from build123d import *

# Parameters (mm, degrees)
F0_W     = 49
F0_H     = 20
F0_W_2   = 5
F0_H_2   = 33
F0_H_3   = 28
F0_H_4   = 5
F0_W_3   = 26.6433528662
F0_W_4   = 30
F0_R     = 3
F1_DEPTH = 3


# Not quite as in the source:
# - a feature names something its author has since deleted; it is built from what else it names


with BuildPart() as f1:
    # F0 (on Front) → F1 (new body)
    with BuildSketch(Plane.XZ):
        with Locations((29.5, 10)):
            Rectangle(F0_W, F0_H)
        with Locations((2.5, 10)):
            Rectangle(F0_W_2, F0_H)
        with Locations((2.5, -16.5)):
            Rectangle(F0_W_2, F0_H_2)
        with Locations((56.5, 10)):
            Rectangle(F0_W_2, F0_H)
        with Locations((56.5, -14)):
            Rectangle(F0_W_2, F0_H_3)
        with Locations((56.5, -30.5)):
            Rectangle(F0_W_2, F0_H_4)
        with Locations((72.3216764331, -14)):
            Rectangle(F0_W_3, F0_H_3)
        with Locations((72.3216764331, 10)):
            Rectangle(F0_W_3, F0_H)
        with Locations((100.6433528662, -14)):
            Rectangle(F0_W_4, F0_H_3)
        with Locations((104, -14)):
            Circle(F0_R, mode=Mode.SUBTRACT)
    extrude(amount=F1_DEPTH)


solid = f1.part
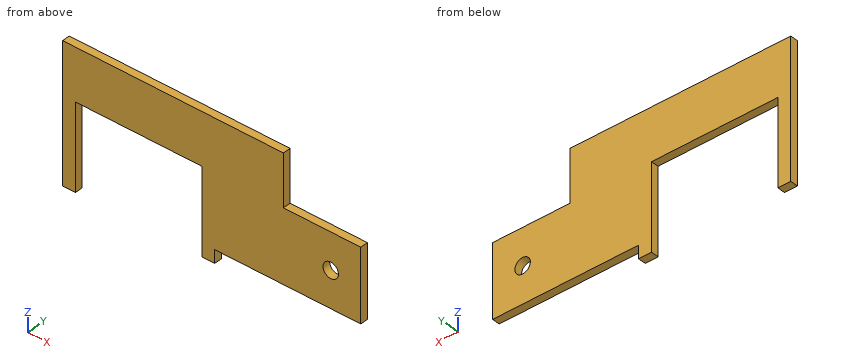
Design review of the part built by this model. Coordinates are the model's own, in mm. Round coordinates to 2 decimals unless told otherwise and drop trailing zeros. Order: outer loops, then holes, each group sorted by start corner. A loop starts at its lowest first (then second) coordinate and runs counter-clockwise, first axis right, second up.
1) Consider section B-B (z = -20). State the section outline as (x, y) points, plus the area to 3 significant figures.
The answers:
outline: (0, -3) - (5, -3) - (5, 0) - (0, 0) - close; (54, -3) - (115.64, -3) - (115.64, 0) - (54, 0) - close
area: 200 mm2
2) Consider section D-D (z = -14). State the section outline as (x, y) points, plus the area to 3 significant figures.
The answers:
outline: (0, -3) - (5, -3) - (5, 0) - (0, 0) - close; (54, -3) - (101, -3) - (101, 0) - (54, 0) - close; (107, -3) - (115.64, -3) - (115.64, 0) - (107, 0) - close
area: 182 mm2
3) Consider section C-C (y = -0.55). State the section outline as (x, z) points, plus the area to 3 significant figures.
The answers:
outline: (0, -33) - (5, -33) - (5, 0) - (54, 0) - (54, -33) - (59, -33) - (59, -28) - (115.64, -28) - (115.64, 0) - (85.64, 0) - (85.64, 20) - (0, 20) - close; hole circle Ø6 at (104, -14)
area: 3,600 mm2
4) Clearance check with flat-ended pins moving along their axes: pin 1 Ø1.5 at (x, y) = (37, -2) entering from -Z; pin 2 Ø0.9 at (y, z) = (-1, 12.5) entering from +X; pin 3 Ø10 at (x, z) = (72, 9.5) entering from +Y. State where each tip first meets the part, or that it passes through.
The answers:
pin 1: stops at z = 0
pin 2: stops at x = 85.64
pin 3: stops at y = 0
5) For L1, parallel to Z at x = 104, y = -1.55; L2, parallel to X at y = -1.95, z = -18; L3, parallel to X at y = -0.35, z = -31, list the stretches that pass through material, from the lowest coordinate up.
The answers:
L1: z = -28 to -17, -11 to 0
L2: x = 0 to 5, 54 to 115.64
L3: x = 0 to 5, 54 to 59
6) Consider section A-A (x = 104). State the section outline as (y, z) points, plus the area to 3 significant figures.
The answers:
outline: (-3, -28) - (0, -28) - (0, -17) - (-3, -17) - close; (-3, -11) - (0, -11) - (0, 0) - (-3, 0) - close
area: 66.0 mm2
